Read the model definition and answer for the solid it produces. Units are mm, in the model's axes. Face numbers are marked on the shaded views. A direction names the side the tool comes from. Round coordinates to 2 decimals unless told otherwise and drop trailing zeros. Write each loop counter-clockwise with the first axis right and the second up, starting at its lowest first coordinate (ties: lowest second). Pieces come first, ordered by that corner, then holes. Notation, with made-up numbers: (7, 10.5) - (53, 10.5) arc R21 cw to (53, 20.5) - close; hole circle Ø9 at (73, -4). An arc over 180 degrees is marked (long way). One line per item, written item: value. Start each with the question number.
(1) A cutting plane is placed at D-D, the plane y = 1.5. Determine the outline of the cut face in (x, z).
(2) The mould has two halves that part along Y. Classify the marked faces 5, 6 and 7: +Y half, -Y half, draft (parallel to the pull), parting line (faces both ways), or undercut.
(3) A cutting plane is placed at C-C, the plane x = 2.5. Determine the outline of the cut face in (y, z), plus the area to 3 significant figures.
(4) For the marked faces 1, 2, 3 and 4, determine the directions among +Z, -Z, +X, -X, +Y, -Y from which every point of the face is accessible in a straight line to the end or side of a thin tool.
(5) A cutting plane is placed at A-A, the plane z = -5.5. Determine the outline of the cut face in (x, y), plus the area to 4 significant figures.
(6) A cutting plane is placed at B-B, the plane z = 2.5. State how many separate pieces and enclosed holes the cut face has, plus the area to 3 significant figures.
(7) Find the intervals of material crossed by L1, parallel to Y at x = 4.25, z = -10.25; L2, parallel to Y at x = 2.5, z = -1.55; L3, parallel to Z at x = 0.75, y = -7, in increasing order.
(8) Flat-ended cylindrical pins translate along their axes: pin 1 Ø2 at (x, z) = (1, 3.5) entering from -Y; pin 2 Ø1.5 at (x, z) = (4, -10.5) entering from -Y; pin 3 Ø0.9 at (x, z) = (3.5, 3.5) entering from +Y; pin 4 Ø6 at (y, z) = (3, 1) entering from +X. Find the tip coordinate at first contact, or state that the pin passes through.
from build123d import *

# Parameters (mm, degrees)
SKETCH1_W                = 29
SKETCH1_H                = 28
SKETCH1_R                = 1
BOSS_EXTRUDE1_DEPTH      = 2
SKETCH2_W                = 29
SKETCH2_H                = 28
SKETCH2_W_2              = 26.5
SKETCH2_H_2              = 25.5
BOSS_EXTRUDE2_DEPTH      = 3
FILLET1_R                = 1
BOSS_EXTRUDE3_DEPTH      = 2.5
BOSS_EXTRUDE3_DEPTH_BACK = 7.5
SKETCH3_W                = 6
SKETCH3_H                = 8
CHAMFER1_SIZE            = 1.25
CUT_EXTRUDE1_DEPTH       = 32.990000884
CUT_EXTRUDE1_DEPTH_BACK  = 32.990000884
SKETCH5_R                = 1.6
SKETCH7_W                = 3
SKETCH7_H                = 16.5
CUT_EXTRUDE2_DEPTH       = 39.40215359
CHAMFER2_SIZE            = 2
CHAMFER3_SIZE            = 1


with BuildPart() as part:
    # Sketch1 → Boss-Extrude1 (new body)
    with BuildSketch(Plane(origin=(0, 0, 0), x_dir=(0, 0, -1), z_dir=(1, 0, 0))):
        with Locations((-0.022840642, -3.707200481)):
            Rectangle(SKETCH1_W, SKETCH1_H)
        with BuildLine():
            ThreePointArc((-12.522840642, 5.262023113), (-8.931850385, 4.701809261), (-9.492064236, 8.292799519))
            Line((-9.492064236, 8.292799519), (9.446382951, 8.292799519))
            ThreePointArc((9.446382951, 8.292799519), (8.8861691, 4.701809261), (12.477159358, 5.262023113))
            Line((12.477159358, 5.262023113), (12.477159358, -5.176424074))
            ThreePointArc((12.477159358, -5.176424074), (8.227159358, -6.207200481), (12.477159358, -7.237976887))
            Line((12.477159358, -7.237976887), (12.477159358, -15.707200481))
            Line((12.477159358, -15.707200481), (-12.522840642, -15.707200481))
            Line((-12.522840642, -15.707200481), (-12.522840642, -7.237976887))
            ThreePointArc((-12.522840642, -7.237976887), (-8.272840642, -6.207200481), (-12.522840642, -5.176424074))
            Line((-12.522840642, -5.176424074), (-12.522840642, 5.262023113))
        make_face(mode=Mode.SUBTRACT)
        with Locations((-10.522840642, 6.292799519)):
            Circle(SKETCH1_R, mode=Mode.SUBTRACT)
        with Locations((-10.522840642, -6.207200481)):
            Circle(SKETCH1_R, mode=Mode.SUBTRACT)
        with Locations((10.477159358, -6.207200481)):
            Circle(SKETCH1_R, mode=Mode.SUBTRACT)
        with Locations((10.477159358, 6.292799519)):
            Circle(SKETCH1_R, mode=Mode.SUBTRACT)
    extrude(amount=BOSS_EXTRUDE1_DEPTH)

    # Sketch2 → Boss-Extrude2 (add)
    with BuildSketch(Plane(origin=(2, 0, 0), x_dir=(0, 0, -1), z_dir=(1, 0, 0))):
        with Locations((-0.022840642, -3.707200481)):
            Rectangle(SKETCH2_W, SKETCH2_H)
        with Locations((-0.022840642, -3.707200481)):
            Rectangle(SKETCH2_W_2, SKETCH2_H_2, mode=Mode.SUBTRACT)
    extrude(amount=BOSS_EXTRUDE2_DEPTH)

    # Fillet1
    fillet1_edges = [part.edges().sort_by_distance(p)[0] for p in [
        (1, 5.262023113, 12.522840642),
        (1, -5.176424074, 12.522840642),
        (1, -7.237976887, 12.522840642),
        (1, -7.237976887, -12.477159358),
        (1, -5.176424074, -12.477159358),
        (1, 5.262023113, -12.477159358),
        (1, 8.292799519, -9.446382951),
        (1, 8.292799519, 9.492064236),
    ]]
    fillet(fillet1_edges, radius=FILLET1_R)

    # Sketch3 → Boss-Extrude3 (add, two sides: drawn at the far end of the back side and taken through both)
    with BuildSketch(Plane.ZY.offset(-BOSS_EXTRUDE3_DEPTH_BACK)):
        with Locations((0.022840642, -21.707200481)):
            Rectangle(SKETCH3_W, SKETCH3_H)
    extrude(amount=BOSS_EXTRUDE3_DEPTH + BOSS_EXTRUDE3_DEPTH_BACK)

    # Chamfer1
    chamfer1_edges = [part.edges().sort_by_distance(p)[0] for p in [
        (2.5, -25.707200481, -2.977159358),
        (-2.5, -17.707200481, 0.022840642),
        (-2.5, -21.707200481, 3.022840642),
        (-2.5, -21.707200481, -2.977159358),
        (-2.5, -25.707200481, 0.022840642),
        (2.5, -25.707200481, 3.022840642),
        (7.5, -25.707200481, 0.022840642),
        (7.5, -21.707200481, 3.022840642),
        (7.5, -17.707200481, 0.022840642),
        (7.5, -21.707200481, -2.977159358),
        (5, -17.707200481, 0.022840642),
        (0, -17.707200481, 0.022840642),
    ]]
    chamfer(chamfer1_edges, length=CHAMFER1_SIZE - 0.0001)  # a hair under: the kernel refuses the full size

    # Sketch5 → Cut-Extrude1 (cut, two sides: drawn at the far end of the back side and taken through both)
    with BuildSketch(Plane(origin=(0, 0, -2.977159358), x_dir=(-1, 0, 0), z_dir=(0, 0, -1)).offset(-CUT_EXTRUDE1_DEPTH_BACK)):
        with Locations(Location((-2.5, -21.707200481, 0), (0, 0, 90))):
            Circle(SKETCH5_R)
    extrude(amount=CUT_EXTRUDE1_DEPTH + CUT_EXTRUDE1_DEPTH_BACK, mode=Mode.SUBTRACT)

    # Sketch7 → Cut-Extrude2 (cut, through all)
    with BuildSketch(Plane.XZ.offset(-9.042799519)):
        with Locations((3.5, 0.022840642)):
            Rectangle(SKETCH7_W, SKETCH7_H)
    extrude(amount=-CUT_EXTRUDE2_DEPTH, mode=Mode.SUBTRACT)

    # Chamfer2
    chamfer2_edges = [part.edges().sort_by_distance(p)[0] for p in [
        (5, 9.667799519, 8.272840642),
        (5, 9.667799519, -8.227159358),
    ]]
    chamfer(chamfer2_edges, length=CHAMFER2_SIZE)

    # Chamfer3
    chamfer3_edges = [part.edges().sort_by_distance(p)[0] for p in [
        (2.5, 10.292799519, -14.477159358),
        (2.5, -17.707200481, -14.477159358),
        (2.5, -17.707200481, 14.522840642),
        (2.5, 10.292799519, 14.522840642),
    ]]
    chamfer(chamfer3_edges, length=CHAMFER3_SIZE)


solid = part.part
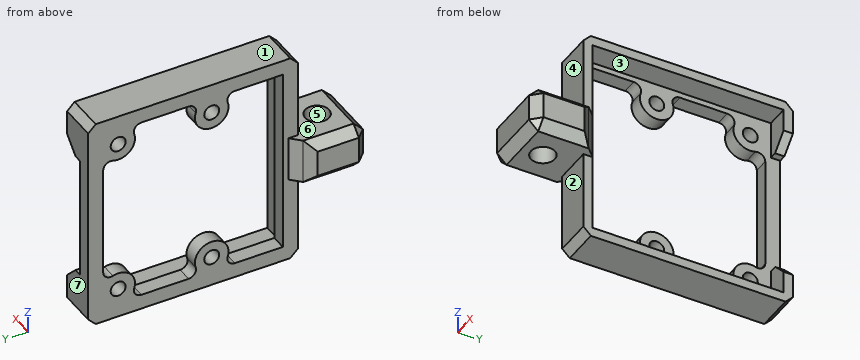
Here are the results:
1. outline: (0, -14.48) - (5, -14.48) - (5, -13.23) - (2, -13.23) - (2, -12.48) - (0, -12.48) - close; (0, 12.52) - (2, 12.52) - (2, 13.27) - (5, 13.27) - (5, 14.52) - (0, 14.52) - close
2. face 5: undercut
2. face 6: draft
2. face 7: +Y half
3. outline: (-25.71, -1.73) - (-24.46, -2.98) - (-23.31, -2.98) - (-23.31, 3.02) - (-24.46, 3.02) - (-25.71, 1.77) - close; (-20.11, -2.98) - (-17.71, -2.98) - (-17.71, -13.48) - (-16.71, -14.48) - (9.29, -14.48) - (10.29, -13.48) - (10.29, -8.23) - (9.04, -8.23) - (9.04, -13.23) - (-16.46, -13.23) - (-16.46, 13.27) - (9.04, 13.27) - (9.04, 8.27) - (10.29, 8.27) - (10.29, 13.52) - (9.29, 14.52) - (-16.71, 14.52) - (-17.71, 13.52) - (-17.71, 3.02) - (-20.11, 3.02) - close
3. area: 141 mm²
4. face 1: +Z, +X, -X, +Y, -Y
4. face 2: -Z, +X, -X, -Y
4. face 3: +X
4. face 4: +Z, +X, -X, -Y
5. outline: (0, -17.71) - (5, -17.71) - (5, -16.46) - (2, -16.46) - (2, -15.71) - (0, -15.71) - close; (0, 8.29) - (2, 8.29) - (2, 10.29) - (0, 10.29) - close
5. area: 11.75 mm²
6. separate pieces: 2
6. enclosed holes: 1
6. area: 66.9 mm²
7. L1: -17.71 to -16.46, 9.04 to 10.29
7. L2: -25.71 to -23.31, -20.11 to -16.46
7. L3: -14.48 to -11.09, -9.87 to -8.37, 8.42 to 9.91, 11.13 to 14.52
8. pin 1: y = -24.98
8. pin 2: y = -17.71
8. pin 3: y = -16.46
8. pin 4: through
